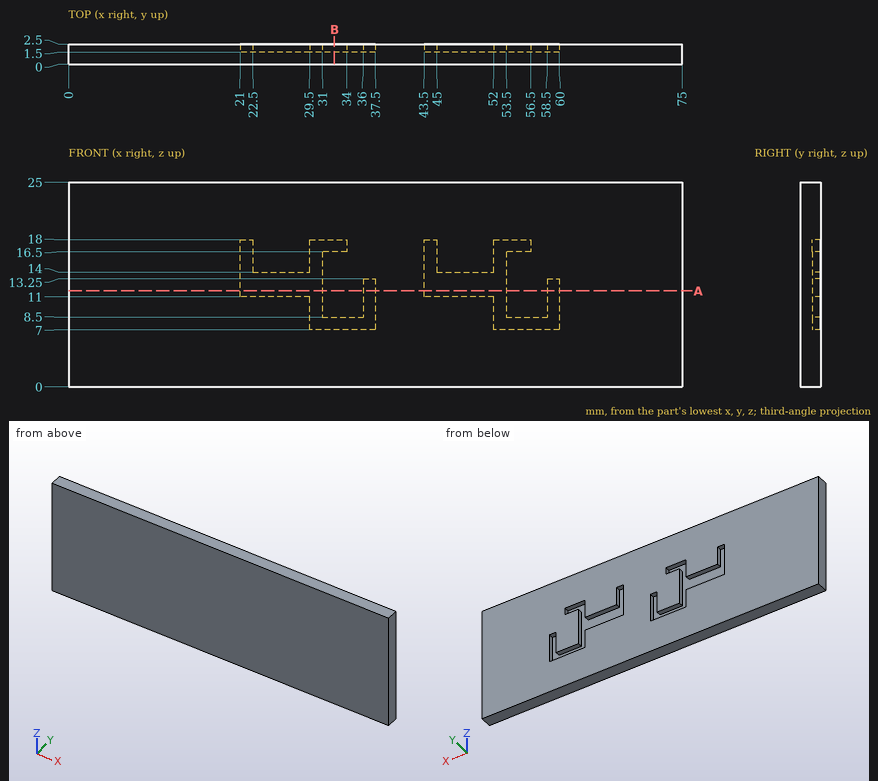
Can you work these out from the drawing? Everything is in mm from the part's minimum corner. Coordinates: 2 decimals unless noted, no trailing zeros. Write each loop counter-clockwise with the first axis right and the second up, starting at its lowest first coordinate (ties: lowest second). Pieces come first, ordered by that corner, then holes. Notation, with made-up numbers: (81, -11.5) -> (104, -11.5) arc R16 ccw to (104, 15.5) -> close; hole circle Ø5 at (22, -35.75). An arc over 180 degrees is marked (long way). Write each question's results on one line, items separated by ' | '. Start each with the question number.
Q1. Imagine slicing it at B-B (x = 32.5). Write out the boundary of the cut face in (y, z), then the cut area to 3 significant figures.
Q2. If I drill on probe 1 along Z at (x, y) = (32, 2.15); probe 2 along Z at (x, y) = (51.5, 1.6), over which ranges is the centre line in solid material (lowest first)?
Q3. Imagine slicing it at A-A (z = 11.75). Write out the boundary of the cut face in (x, y).
Taken from the geometry:
1) outline: (0, 0) -> (2.5, 0) -> (2.5, 7) -> (1.5, 7) -> (1.5, 8.5) -> (2.5, 8.5) -> (2.5, 16.5) -> (1.5, 16.5) -> (1.5, 18) -> (2.5, 18) -> (2.5, 25) -> (0, 25) -> close | area: 59.5 mm^2
2) probe 1: z = 0 to 7, 8.5 to 16.5, 18 to 25 | probe 2: z = 0 to 11, 14 to 25
3) outline: (0, 0) -> (75, 0) -> (75, 2.5) -> (60, 2.5) -> (60, 1.5) -> (58.5, 1.5) -> (58.5, 2.5) -> (53.5, 2.5) -> (53.5, 1.5) -> (43.5, 1.5) -> (43.5, 2.5) -> (37.5, 2.5) -> (37.5, 1.5) -> (36, 1.5) -> (36, 2.5) -> (31, 2.5) -> (31, 1.5) -> (21, 1.5) -> (21, 2.5) -> (0, 2.5) -> close
